Read the model definition and answer for the solid it produces. Units are mm, in the model's axes. Face numbers are marked on the shaded views. Round coordinates to 2 decimals unless told otherwise and drop trailing zeros. Loops run counter-clockwise (first coordinate to the right, second up) from the corner with the lowest first, then second, coordinate; pieces in that order, holes last. Notation, with made-up numbers: (17.25, -6.75) - (38.25, -6.75) arc R14 ccw to (38.25, 18.25) - close; hole circle Ø1 at (4, 79). An arc over 180 degrees is marked (long way). Use CSV: the item, a comma, the result in double quotes. Start each with the question number.
1. Determine the mould class of the marked faces 1, 2 and 3 for opening direction Z: +Z half, -Z half, draft (parallel to the pull), parting line (faces both ways), or undercut.
2. Consider line 1 along Z through (x, y) = (2.15, 12.5); line 2 along Z through (x, y) = (1.75, 9.5); line 3 along X through (y, z) = (12, 11). Determine where each line is inside the solid, lowest interval first.
3. Given pin 1 Ø1.5 at (x, y) = (1, 7) entering from +Z; pin 2 Ø5 at (y, z) = (9.98, -30.24) entering from +X; pin 3 Ø1.5 at (x, y) = (1.5, 11) entering from +Z, each flat-ended and moving along its own axis, determine where each tip first touches the part or whether it passes through.
4. Find section D-D (z = 8). Give the vertices of the cut face in (x, y), and give its area (3 significant figures).
5. Find section B-B (y = 10.75). Give the vertices of the cut face in (x, z), and give its area (3 significant figures).
6. Find section C-C (z = -29.5). Give the vertices of the cut face in (x, y), and give its area (3 significant figures).
7. Find section A-A (x = 0.65). Give the vertices of the cut face in (y, z) (3 decimals).
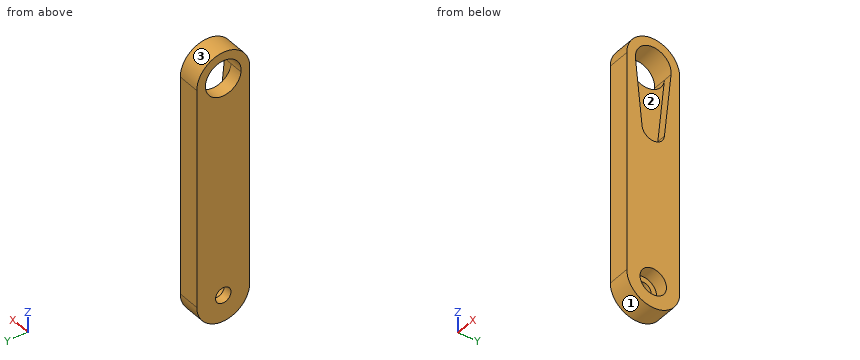
Autodesk Inventor part; units mm, degrees
ref_plane "YZ Plane" through (0, 0, 0) normal (1, 0, 0) x (0, 1, 0)
ref_plane "XZ Plane" through (0, 0, 0) normal (0, 1, 0) x (-1, 0, 0)
ref_plane "XY Plane" through (0, 0, 0) normal (0, 0, 1) x (1, 0, 0)
sketch "Szkic1" plane through (0, 0, 0) normal (1, 0, 0) x (0, 1, 0)
  line L0 (9.9771, 19.755) -> (9.9771, -30.245) construction
  line L1 (3.9771, 19.755) -> (3.9771, -30.245)
  line L2 (15.9771, -30.245) -> (15.9771, 19.755)
  arc A0 (15.9771, 19.755) -> (3.9771, 19.755) centre (9.9771, 19.755) ccw
  arc A1 (3.9771, -30.245) -> (15.9771, -30.245) centre (9.9771, -30.245) ccw
  circle A2 centre (9.9771, 19.755) radius 1.6
  circle A3 centre (9.9771, -30.245) radius 1.75
  point P0 (0, 0)
  point P1 (9.9771, -5.245)
  dimension "d0" = 50
  dimension "d1" = 12
  dimension "d2" = 3.2
  dimension "d3" = 3.5
extrude "Wyciągnięcie proste1" add sketch "Szkic1" along normal blind 3
sketch "Szkic4" plane through (3, 0, 0) normal (1, 0, 0) x (0, 0, -1)
  circle A0 centre (-19.755, 9.9771) radius 1.6
  arc A1 (-19.38, 13.7083) -> (-19.38, 6.2459) centre (-19.755, 9.9771) ccw
  arc A2 (-4.53, 7.7383) -> (-4.53, 12.2158) centre (-4.755, 9.9771) ccw
  line L0 (-19.38, 13.7083) -> (-4.53, 12.2158)
  line L1 (-19.38, 6.2459) -> (-4.53, 7.7383)
  line L2 (-4.5, 12.5143) -> (-19.35, 14.0068)
  arc A3 (-19.35, 14.0068) -> (-19.35, 5.9474) centre (-19.755, 9.9771) ccw
  line L3 (-19.35, 5.9474) -> (-4.5, 7.4398)
  arc A4 (-4.5, 7.4398) -> (-4.5, 12.5143) centre (-4.755, 9.9771) ccw
  circle A5 centre (-19.755, 9.9771) radius 4.05
  arc A6 (30.245, 3.9771) -> (30.245, 15.9771) centre (30.245, 9.9771) ccw
  line L4 (30.245, 15.9771) -> (-19.755, 15.9771)
  arc A7 (-19.755, 15.9771) -> (-19.755, 3.9771) centre (-19.755, 9.9771) ccw
  line L5 (-19.755, 3.9771) -> (30.245, 3.9771)
  circle A8 centre (30.245, 9.9771) radius 1.75
  circle A9 centre (-19.755, 9.9771) radius 1.6
  point P0 (0, 0)
  point P1 (-19.35, 14.0068)
  dimension "d12" = 7.5
  dimension "d13" = 4.5
  dimension "d14" = 15
  dimension "d15" = 0.3
extrude "Wyciągnięcie proste4" add sketch "Szkic4" along normal blind 2 contours L5 A7 L4 A6
extrude "Wyciągnięcie proste5" cut sketch "Szkic4" against normal blind 3 contours A0 | L0 A5 L1 A1 | A1 L1 A5 A3 L0
sketch "Szkic5" plane through (5, 0, 0) normal (1, 0, 0) x (0, 0, -1)
  circle A0 centre (30.245, 9.9771) radius 1.75
  circle A1 centre (30.245, 9.9771) radius 3
  point P0 (0, 0)
  dimension "d20" = 6
extrude "Wyciągnięcie proste6" cut sketch "Szkic5" against normal blind 3 contours A0 | A1
properties part number "belka"
Filled sheet:
1,face 1,"-Z half"
1,face 2,"undercut"
1,face 3,"+Z half"
2,line 1,"z = -35.69 to -31.87, -28.62 to 16.59, 22.92 to 25.2"
2,line 2,"z = -36.23 to -31.93, -28.56 to 15.73, 23.78 to 25.74"
2,line 3,"x = 0 to 3"
3,pin 1,"stops at z = 25.33"
3,pin 2,"stops at x = 2"
3,pin 3,"stops at z = 25.75"
4,outline,"(0, 3.98) - (5, 3.98) - (5, 7.09) - (3, 7.09) - (3, 12.87) - (5, 12.87) - (5, 15.98) - (0, 15.98) - close"
4,area,"48.4 mm²"
5,outline,"(0, -36.2) - (5, -36.2) - (5, -33.14) - (2, -33.14) - (2, -31.82) - (0, -31.82) - close; (0, -28.67) - (2, -28.67) - (2, -27.35) - (5, -27.35) - (5, 2.32) - (3, 2.32) - (3, 15.78) - (0, 15.78) - close; (0, 23.73) - (5, 23.73) - (5, 25.71) - (0, 25.71) - close"
5,area,"219 mm²"
6,outline,"(0, 3.98) - (5, 3.98) - (5, 7.07) - (2, 7.07) - (2, 8.39) - (0, 8.39) - close; (0, 11.56) - (2, 11.56) - (2, 12.88) - (5, 12.88) - (5, 15.98) - (0, 15.98) - close"
6,area,"36.2 mm²"
7,outline,"(3.977, -30.245) arc R6 ccw to (15.977, -30.245) - (15.977, 19.755) arc R6 ccw to (3.977, 19.755) - close; hole (5.947, 19.35) arc R4.05 ccw to (14.007, 19.35) arc R4.05 ccw (long way) to start; hole circle Ø3.5 at (9.977, -30.245)"
